Geometry check sheet. Reference: the model listing, model coordinates, mm. Face numbers are marked on the shaded views. Give positions to 0.01 mm unless a question says otherwise; leave off trailing zeros. Write each loop counter-clockwise with the first axis right and the second up, starting at its lowest first coordinate (ties: lowest second). Pieces come first, ordered by that corner, then holes. Notation, with made-up numbers: (51.5, 29) - (79.5, 29) arc R34 ccw to (79.5, 61) - close; hole circle Ø8 at (-27.75, 52.5). An arc over 180 degrees is marked (long way). Use a Markdown table: item, result.
```python
from build123d import *

# Parameters (mm, degrees)
SKETCH1_W           = 52
SKETCH1_H           = 20
BOSS_EXTRUDE1_DEPTH = 2
SKETCH2_R           = 3
SKETCH2_R_2         = 1.5
BOSS_EXTRUDE2_DEPTH = 4
SKETCH3_R           = 1.5
CUT_EXTRUDE1_DEPTH  = 56.856960175
FILLET1_R           = 2


with BuildPart() as part:
    # Sketch1 → Boss-Extrude1 (new body)
    with BuildSketch(Plane(origin=(0, 0, 0), x_dir=(1, 0, 0), z_dir=(0, 1, 0))):
        with Locations((26, 10)):
            Rectangle(SKETCH1_W, SKETCH1_H)
    extrude(amount=BOSS_EXTRUDE1_DEPTH)

    # Sketch2 → Boss-Extrude2 (add)
    # profile 1 of 4: a face of its own
    with BuildSketch(Plane(origin=(0, 2, 0), x_dir=(1, 0, 0), z_dir=(0, 1, 0))):
        with Locations(Location((5, 16.25, 0), (0, 0, 90))):
            Circle(SKETCH2_R)
        with Locations(Location((5, 16.25, 0), (0, 0, 270))):
            Circle(SKETCH2_R_2, mode=Mode.SUBTRACT)
    # profile 2 of 4: a face of its own
    with BuildSketch(Plane(origin=(0, 2, 0), x_dir=(1, 0, 0), z_dir=(0, 1, 0))):
        with Locations(Location((5, 3.75, 0), (0, 0, 90))):
            Circle(SKETCH2_R)
        with Locations(Location((5, 3.75, 0), (0, 0, 270))):
            Circle(SKETCH2_R_2, mode=Mode.SUBTRACT)
    # profile 3 of 4: a face of its own
    with BuildSketch(Plane(origin=(0, 2, 0), x_dir=(1, 0, 0), z_dir=(0, 1, 0))):
        with Locations(Location((47, 3.75, 0), (0, 0, 90))):
            Circle(SKETCH2_R)
        with Locations(Location((47, 3.75, 0), (0, 0, 270))):
            Circle(SKETCH2_R_2, mode=Mode.SUBTRACT)
    # profile 4 of 4: a face of its own
    with BuildSketch(Plane(origin=(0, 2, 0), x_dir=(1, 0, 0), z_dir=(0, 1, 0))):
        with Locations(Location((47, 16.25, 0), (0, 0, 90))):
            Circle(SKETCH2_R)
        with Locations(Location((47, 16.25, 0), (0, 0, 270))):
            Circle(SKETCH2_R_2, mode=Mode.SUBTRACT)
    extrude(amount=BOSS_EXTRUDE2_DEPTH)

    # Sketch3 → Cut-Extrude1 (cut, through all)
    with BuildSketch(Plane(origin=(0, 2, 0), x_dir=(1, 0, 0), z_dir=(0, 1, 0))):
        with Locations(Location((47, 3.75, 0), (0, 0, 270))):
            Circle(SKETCH3_R)
        with Locations(Location((47, 16.25, 0), (0, 0, 270))):
            Circle(SKETCH3_R)
        with Locations(Location((5, 3.75, 0), (0, 0, 270))):
            Circle(SKETCH3_R)
        with Locations(Location((5, 16.25, 0), (0, 0, 270))):
            Circle(SKETCH3_R)
    extrude(amount=-CUT_EXTRUDE1_DEPTH, mode=Mode.SUBTRACT)

    # Fillet1
    fillet1_edges = [part.edges().sort_by_distance(p)[0] for p in [
        (0, 1, -20),
        (52, 1, -20),
        (52, 1, 0),
        (0, 1, 0),
    ]]
    fillet(fillet1_edges, radius=FILLET1_R)


solid = part.part
```
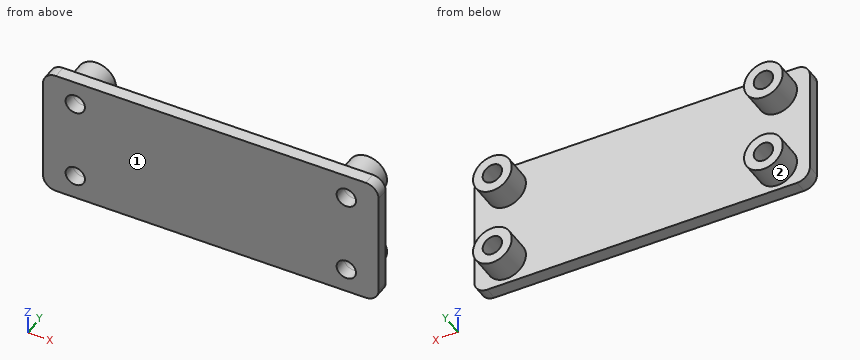
1) Material ranges on L1, parallel to X at y = 1.4, z = -16.25; L2, parallel to X at y = 5.25, z = -16.25; L3, parallel to X at y = 0.4, z = -17.25, recorded low to high. Write a range as from..to.
Working result:
| item | result |
|---|---|
| L1 | x = 0..3.5, 6.5..45.5, 48.5..52 |
| L2 | x = 2..3.5, 6.5..8, 44..45.5, 48.5..50 |
| L3 | x = 0..3.88, 6.12..45.88, 48.12..52 |
2) Section check C-C on z = -3.75. Record the boundary of the cut face in (x, y), then the cut area to 3 significant figures.
Working result:
| item | result |
|---|---|
| outline | (0, 0) - (3.5, 0) - (3.5, 6) - (2, 6) - (2, 2) - (0, 2) - close; (6.5, 0) - (45.5, 0) - (45.5, 6) - (44, 6) - (44, 2) - (8, 2) - (8, 6) - (6.5, 6) - close; (48.5, 0) - (52, 0) - (52, 2) - (50, 2) - (50, 6) - (48.5, 6) - close |
| area | 116 mm² |
3) Section check D-D on y = 1.4. Record the boundary of the cut face in (x, z).
Working result:
| item | result |
|---|---|
| outline | (0, -18) arc R2 ccw to (2, -20) - (50, -20) arc R2 ccw to (52, -18) - (52, -2) arc R2 ccw to (50, 0) - (2, 0) arc R2 ccw to (0, -2) - close; hole circle Ø3 at (5, -16.25); hole circle Ø3 at (5, -3.75); hole circle Ø3 at (47, -16.25); hole circle Ø3 at (47, -3.75) |
4) Section check B-B on x = 5. Record the boundary of the cut face in (y, z).
Working result:
| item | result |
|---|---|
| outline | (0, -20) - (2, -20) - (2, -19.25) - (6, -19.25) - (6, -17.75) - (0, -17.75) - close; (0, -14.75) - (6, -14.75) - (6, -13.25) - (2, -13.25) - (2, -6.75) - (6, -6.75) - (6, -5.25) - (0, -5.25) - close; (0, -2.25) - (6, -2.25) - (6, -0.75) - (2, -0.75) - (2, 0) - (0, 0) - close |
5) Depth check by flat-ended pin: P1, Ø2, axis at x = 20.5, z = -9.5, coming from the +Y side; P2, Ø2.5, axis at x = 5, z = -16.25, coming from the +Y side; P3, Ø1, axis at y = 3.5, z = -17.5, coming from the +X side; P4, Ø3, axis at y = 4, z = -17.5, coming from the +X side. Enter the tip coordinate at first touch or a pass-through.
Working result:
| item | result |
|---|---|
| P1 | stops at y = 2 |
| P2 | passes through |
| P3 | stops at x = 49.9 |
| P4 | stops at x = 50 |
6) Mould release check, pull along X, two halves, no side actions. Record for the marked faces 1 and 2: pulls with the +X half, pulls with the -X half, needs draft (parallel to the pull), parting line crosses it, or undercut.
Working result:
| item | result |
|---|---|
| face 1 | needs draft |
| face 2 | undercut |
7) Section check A-A on y = 5.5. Record the boundary of the cut face in (x, z), then the cut area to 3 significant figures.
Working result:
| item | result |
|---|---|
| outline | circle Ø6 at (5, -16.25); circle Ø6 at (5, -3.75); circle Ø6 at (47, -16.25); circle Ø6 at (47, -3.75); hole circle Ø3 at (5, -16.25); hole circle Ø3 at (5, -3.75); hole circle Ø3 at (47, -16.25); hole circle Ø3 at (47, -3.75) |
| area | 84.8 mm² |
